```python
from build123d import *

# Parameters (mm, degrees)
BOSS_EXTRUDE1_DEPTH = 12.7
CUT_EXTRUDE5_DEPTH  = 12.7
SKETCH9_R           = 3.81
CUT_EXTRUDE6_DEPTH  = 2.54
CUT_EXTRUDE7_DEPTH  = 12.7


with BuildPart() as part:
    # Sketch1 → Boss-Extrude1 (new body)
    with BuildSketch(Plane.XY.offset(1081.90385267)):
        with BuildLine():
            Line((779.192327096, 749.508856284), (760.142327096, 749.508856284))
            Line((760.142327096, 749.508856284), (477.497001613, 586.250864284))
            Line((477.497001613, 586.250864284), (477.497001613, 557.307056284))
            ThreePointArc((477.497001613, 557.307056284), (392.915001613, 472.725056284), (308.333001613, 557.307056284))
            Line((308.333001613, 557.307056284), (308.289027096, 586.225464284))
            Line((308.289027096, 586.225464284), (25.599727096, 749.508856284))
            Line((25.599727096, 749.508856284), (6.549727096, 749.508856284))
            Line((6.549727096, 749.508856284), (6.549727096, 162.006856284))
            Line((6.549727096, 162.006856284), (779.192327096, 162.006856284))
            Line((779.192327096, 162.006856284), (779.192327096, 749.508856284))
        make_face()
    extrude(amount=-BOSS_EXTRUDE1_DEPTH)

    # Sketch7 → Cut-Extrude5 (cut)
    with BuildSketch(Plane(origin=(0, 0, 1069.20385267), x_dir=(-1, 0, 0), z_dir=(0, 0, -1))):
        with BuildLine():
            Line((-424.665001613, 346.156856284), (-361.165001613, 346.156856284))
            ThreePointArc((-361.165001613, 346.156856284), (-356.674873552, 348.016728223), (-354.815001613, 352.506856284))
            Line((-354.815001613, 352.506856284), (-354.815001613, 416.006856284))
            ThreePointArc((-354.815001613, 416.006856284), (-356.674873552, 420.496984344), (-361.165001613, 422.356856284))
            Line((-361.165001613, 422.356856284), (-424.665001613, 422.356856284))
            ThreePointArc((-424.665001613, 422.356856284), (-429.155129673, 420.496984344), (-431.015001613, 416.006856284))
            Line((-431.015001613, 416.006856284), (-431.015001613, 352.506856284))
            ThreePointArc((-431.015001613, 352.506856284), (-429.155129673, 348.016728223), (-424.665001613, 346.156856284))
        make_face()
    extrude(amount=-CUT_EXTRUDE5_DEPTH, mode=Mode.SUBTRACT)

    # Sketch9 → Cut-Extrude6 (cut)
    with BuildSketch(Plane(origin=(0, 0, 1069.20385267), x_dir=(-1, 0, 0), z_dir=(0, 0, -1))):
        with Locations((-466.165162315, 515.016056284)):
            Circle(SKETCH9_R)
        with Locations((-319.66484091, 515.016056284)):
            Circle(SKETCH9_R)
    extrude(amount=-CUT_EXTRUDE6_DEPTH, mode=Mode.SUBTRACT)

    # Sketch10 → Cut-Extrude7 (cut)
    with BuildSketch(Plane(origin=(0, 0, 1069.20385267), x_dir=(-1, 0, 0), z_dir=(0, 0, -1))):
        with BuildLine():
            Line((-82.919210129, 701.800959598), (-118.114482539, 681.480959598))
            ThreePointArc((-118.114482539, 681.480959598), (-120.438743853, 672.806698284), (-111.764482539, 670.48243697))
            Line((-111.764482539, 670.48243697), (-76.569210129, 690.80243697))
            ThreePointArc((-76.569210129, 690.80243697), (-74.244948815, 699.476698284), (-82.919210129, 701.800959598))
        make_face()
        with BuildLine():
            Line((-702.910793096, 701.800959598), (-667.715520686, 681.480959598))
            ThreePointArc((-667.715520686, 681.480959598), (-665.391259372, 672.806698284), (-674.065520686, 670.48243697))
            Line((-674.065520686, 670.48243697), (-709.260793096, 690.80243697))
            ThreePointArc((-709.260793096, 690.80243697), (-711.58505441, 699.476698284), (-702.910793096, 701.800959598))
        make_face()
        with BuildLine():
            Line((-153.309754949, 661.160959597), (-188.505027358, 640.840959598))
            ThreePointArc((-188.505027358, 640.840959598), (-190.829288672, 632.166698284), (-182.155027358, 629.84243697))
            Line((-182.155027358, 629.84243697), (-146.959754949, 650.16243697))
            ThreePointArc((-146.959754949, 650.16243697), (-144.635493635, 658.836698283), (-153.309754949, 661.160959597))
        make_face()
        with BuildLine():
            Line((-638.870248276, 650.16243697), (-603.674975867, 629.84243697))
            ThreePointArc((-603.674975867, 629.84243697), (-595.000714553, 632.166698284), (-597.324975867, 640.840959598))
            Line((-597.324975867, 640.840959598), (-632.520248276, 661.160959598))
            ThreePointArc((-632.520248276, 661.160959598), (-641.19450959, 658.836698284), (-638.870248276, 650.16243697))
        make_face()
        with BuildLine():
            Line((-568.479703457, 609.52243697), (-533.284431047, 589.20243697))
            ThreePointArc((-533.284431047, 589.20243697), (-524.610169733, 591.526698284), (-526.934431047, 600.200959598))
            Line((-526.934431047, 600.200959598), (-562.129703457, 620.520959598))
            ThreePointArc((-562.129703457, 620.520959598), (-570.803964771, 618.196698284), (-568.479703457, 609.52243697))
        make_face()
        with BuildLine():
            Line((-223.700299768, 620.520959597), (-258.895572178, 600.200959597))
            ThreePointArc((-258.895572178, 600.200959597), (-261.219833492, 591.526698284), (-252.545572178, 589.20243697))
            Line((-252.545572178, 589.20243697), (-217.350299768, 609.52243697))
            ThreePointArc((-217.350299768, 609.52243697), (-215.026038454, 618.196698283), (-223.700299768, 620.520959597))
        make_face()
    extrude(amount=-CUT_EXTRUDE7_DEPTH, mode=Mode.SUBTRACT)


solid = part.part
```
Work out the finished part from the listing and answer in its coordinate system (mm). A direction names the side the tool comes from. Give positions to 0.01 mm unless a question says otherwise; leave off trailing zeros. Write each loop counter-clockwise with the first axis right and the second up, starting at its lowest first coordinate (ties: lowest second). Pieces come first, ordered by that corner, then holes. Notation, with made-up numbers: (50, 54) -> (61, 54) arc R38 ccw to (61, 92) -> close; hole circle Ø2 at (-34, 70.5). An arc over 180 degrees is marked (long way). Write item = value, one per line.
Q1. Section A-A on x = 615.5 is taken. Determine the outline of the cut face in (y, z).
Computed values:
outline = (162.01, 1069.2) -> (636.67, 1069.2) -> (636.67, 1081.9) -> (162.01, 1081.9) -> close; (651.33, 1069.2) -> (665.96, 1069.2) -> (665.96, 1081.9) -> (651.33, 1081.9) -> close
Q2. Section C-C on z = 1074 is taken. State how many separate pieces and enclosed holes the cut face has, and give its area (3 significant figures).
Computed values:
separate_pieces = 1
enclosed_holes = 7
area = 354,000 mm^2
Q3. A tool of negligible diameter and unlimited length cuts with its end or side. For faces 1 (the flat face through (691.42, 680.5, 1075.46)), 2 (the flat face through (168.923, 666.724, 1075.643)), 3 (the flat face through (387, 460, 1069.204)), from which of +Z, -Z, +X, -X, +Y, -Y can it reach the whole face along a straight path? Write none if from no direction.
Computed values:
face_1 = +Z, -Z
face_2 = +Z, -Z, +Y
face_3 = -Z, +X, -X, +Y, -Y
Q4. Consider line 1 along X through (y, z) = (685, 1078.5); line 2 along X through (y, z) = (607, 1075.5); line 3 along X through (y, z) = (415, 1073.25) (3 decimals). Determine where each line is inside the solid, lowest interval first.
Computed values:
line_1 = 6.55 to 86.62, 112.02 to 137.28, 648.46 to 673.81, 699.21 to 779.19
line_2 = 6.55 to 221.72, 247.12 to 272.32, 513.42 to 538.71, 564.11 to 779.19
line_3 = 6.55 to 354.815, 431.015 to 779.192
Q5. Flat-ended cylindrical pins translate along their axes: pin 1 Ø6.5 at (x, z) = (403, 1075.5) entering from +Y; pin 2 Ø6 at (x, z) = (527.5, 1072) entering from +Y; pin 3 Ø3 at (x, z) = (166.5, 1071.5) entering from +Y. Find the tip coordinate at first contact, or state that the pin passes through.
Computed values:
pin_1 = 473.78
pin_2 = 616.87
pin_3 = 668.99
Q6. Section B-B on y = 486.5 is taken. Determine the outline of the cut face in (x, z), and give its area (3 significant figures).
Computed values:
outline = (6.55, 1069.2) -> (346.65, 1069.2) -> (346.65, 1081.9) -> (6.55, 1081.9) -> close; (439.18, 1069.2) -> (779.19, 1069.2) -> (779.19, 1081.9) -> (439.18, 1081.9) -> close
area = 8,640 mm^2
Q7. Section D-D on x = 508.5 is taken. Determine the outline of the cut face in (y, z).
Computed values:
outline = (162.01, 1069.2) -> (604.16, 1069.2) -> (604.16, 1081.9) -> (162.01, 1081.9) -> close
Q8. For a pull along X with two mould halves and no side action, classify faces 4 (the flat face through (387, 460, 1081.904)), 5 (the flat face through (235.194, 599.22, 1075.465)) as pulls with the +X half, pulls with the -X half, needs draft (parallel to the pull), parting line crosses it, or undercut.
Computed values:
face_4 = needs draft
face_5 = undercut
